from build123d import *

# Parameters (mm, degrees)
BOSS_EXTRU_1_DEPTH      = 4.9
BOSS_EXTRU_1_DEPTH_BACK = 4.9
ESQUISSE1_R             = 1.55
CUT_EXTRUDE1_START      = -2
CUT_EXTRUDE1_DEPTH      = 2
BOSS_EXTRUDE1_START     = 1.8
SKETCH2_R               = 3.55
SKETCH2_R_2             = 1.55
BOSS_EXTRUDE1_DEPTH     = 1.8


with BuildPart() as part:
    # Esquisse1 → Boss.-Extru.1 (new, two sides: drawn at the far end of the back side and taken through both)
    with BuildSketch(Plane.XY.offset(-BOSS_EXTRU_1_DEPTH_BACK)):
        with BuildLine():
            ThreePointArc((-7.035134666, 91.99317437), (-10.542037141, 94.941857654), (-15, 96))
            ThreePointArc((-15, 96), (-19, 100), (-15, 104))
            ThreePointArc((-15, 104), (-5.711685092, 101.40489844), (0.886406153, 94.37122672))
            Line((0.886406153, 94.37122672), (4, 0))
            ThreePointArc((4, 0), (0, -4), (-4, 0))
            Line((-4, 0), (-7.035134666, 91.99317437))
        make_face()
        with Locations((-15, 100)):
            Circle(ESQUISSE1_R, mode=Mode.SUBTRACT)
        Circle(ESQUISSE1_R, mode=Mode.SUBTRACT)
    extrude(amount=BOSS_EXTRU_1_DEPTH + BOSS_EXTRU_1_DEPTH_BACK)

    # Sketch1 → Cut-Extrude1 (cut)
    with BuildSketch(Plane.XY.offset(4.9).offset(CUT_EXTRUDE1_START)):
        with BuildLine():
            Line((-7.035134666, 91.99317437), (-4.166311888, 5.040817029))
            Line((-4.166311888, 5.040817029), (3.833688112, 5.040817029))
            Line((3.833688112, 5.040817029), (0.886406153, 94.37122672))
            ThreePointArc((0.886406153, 94.37122672), (-5.711685092, 101.40489844), (-15, 104))
            ThreePointArc((-15, 104), (-19, 100), (-15, 96))
            ThreePointArc((-15, 96), (-10.542037141, 94.941857654), (-7.035134666, 91.99317437))
        make_face()
    cut_extrude1 = extrude(amount=CUT_EXTRUDE1_DEPTH, mode=Mode.SUBTRACT)

    # Mirror1: Cut-Extrude1 across plane
    add(cut_extrude1.mirror(Plane.XY), mode=Mode.SUBTRACT)

    # Sketch2 → Boss-Extrude1 (add)
    with BuildSketch(Plane(origin=(0, 0, -2.9), x_dir=(-1, 0, 0), z_dir=(0, 0, -1)).offset(BOSS_EXTRUDE1_START)):
        with Locations((15, 100)):
            Circle(SKETCH2_R)
        with Locations(Location((15, 100, 0), (0, 0, 180))):
            Circle(SKETCH2_R_2, mode=Mode.SUBTRACT)
    extrude(amount=-BOSS_EXTRUDE1_DEPTH)


solid = part.part
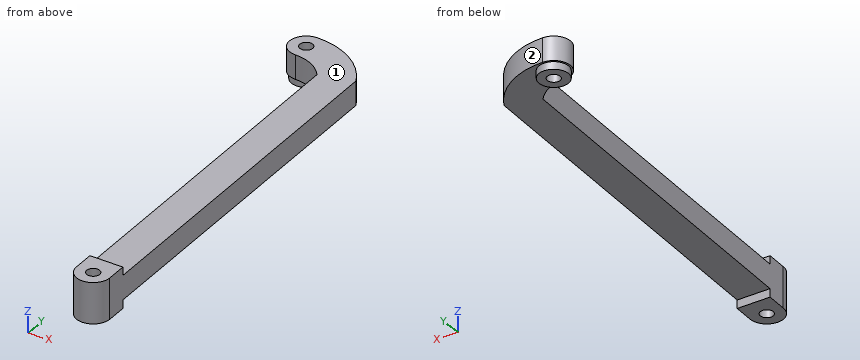
Model file for the job. Use its own axes, mm. Face numbers are marked on the shaded views. A direction names the side the tool comes from. Give positions to 0.01 mm unless a question says otherwise; leave off trailing zeros. Loops run counter-clockwise (first coordinate to the right, second up) from the corner with the lowest first, then second, coordinate; pieces in that order, holes last. Notation, with made-up numbers: (-36.5, 78) -> (-14.5, 78) arc R29 ccw to (-14.5, 114) -> close; hole circle Ø5 at (66, 61.5). An arc over 180 degrees is marked (long way). Use a Markdown table: item, result. Add a question column.
(1) Drop flat-ended pins along their axis: pin 1 Ø4 at (x, y) = (-15, 100) entering from -Z; pin 2 Ø7 at (x, y) = (-6, 78.5) entering from -Z; pin 3 Ø0.6 at (x, z) = (1, 3.5) entering from +Y. Give the stop position or say it passes through.
(2) Slice it at D-D on y = 10. List the corners of the cut face in (x, z), and give its area (3 significant figures).
(3) Slice it at C-C on x = -12.5. List the corners of the cut face in (y, z).
(4) Tool access for the marked faces 1 and 2: list every direction of +Z, -Z, +X, -X, +Y, -Y with a clear straight run to the whole face (end or side of a thin tool).
(5) Slice it at B-B on y = 100. List the corners of the cut face in (x, z).
(6) Wall check: line 1 along Z through (x, y) = (0.5, 33); line 2 along Y through (x, z) = (-15, -1.25); line 3 along Y through (x, z) = (-14.75, -3.5). Give the ranges that are in metal, low to high.
(7) Slice it at A-A on z = -1.75. List the corners of the cut face in (x, y).
Filled sheet:
| question | item | result |
|---|---|---|
| 1 | pin 1 | z = -4.7 |
| 1 | pin 2 | z = -2.9 |
| 1 | pin 3 | y = 5.04 |
| 2 | outline | (-4.33, -2.9) -> (3.67, -2.9) -> (3.67, 2.9) -> (-4.33, 2.9) -> close |
| 2 | area | 46.4 mm2 |
| 3 | outline | (95.68, -2.9) -> (97.48, -2.9) -> (97.48, -4.7) -> (102.52, -4.7) -> (102.52, -2.9) -> (103.82, -2.9) -> (103.82, 2.9) -> (95.68, 2.9) -> close |
| 4 | face 1 | +Z, +X, -X, +Y |
| 4 | face 2 | +Z, -Z, +X, +Y |
| 5 | outline | (-19, -2.9) -> (-18.55, -2.9) -> (-18.55, -4.7) -> (-16.55, -4.7) -> (-16.55, 2.9) -> (-19, 2.9) -> close; (-13.45, -4.7) -> (-11.45, -4.7) -> (-11.45, -2.9) -> (-3.71, -2.9) -> (-3.71, 2.9) -> (-13.45, 2.9) -> close |
| 6 | line 1 | -2.9 to 2.9 |
| 6 | line 2 | 96 to 98.45, 101.55 to 104 |
| 6 | line 3 | 96.46 to 98.47, 101.53 to 103.54 |
| 7 | outline | (-15, 96) arc R9.92 cw to (-7.04, 91.99) -> (-4, 0) arc R4 ccw to (4, 0) -> (0.89, 94.37) arc R17.92 ccw to (-15, 104) arc R4 ccw to start; hole circle Ø3.1 at (-15, 100); hole circle Ø3.1 at (0, 0) |
